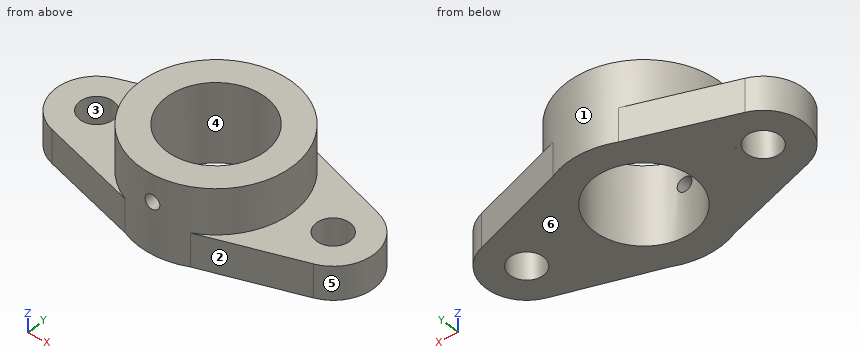
Autodesk Inventor part; units mm, degrees
ref_plane "YZ Plane" through (0, 0, 0) normal (1, 0, 0) x (0, 1, 0)
ref_plane "XZ Plane" through (0, 0, 0) normal (0, 1, 0) x (-1, 0, 0)
ref_plane "XY Plane" through (0, 0, 0) normal (0, 0, 1) x (1, 0, 0)
sketch "Boceto1" plane through (0, 0, 0) normal (0, 0, 1) x (1, 0, 0)
  circle A0 centre (-27.7266, -0.9426) radius 7
  circle A1 centre (-20, 3.239) radius 0.1677
  circle A2 centre (68.2698, -0.1077) radius 7
  arc A3 (73.4655, -16.2943) -> (73.5445, 16.0533) centre (68.2698, -0.1077) ccw
  circle A4 centre (20.2642, 0) radius 32
  line L0 (-33.3043, 15.1163) -> (6.9422, 29.0951)
  line L1 (73.5445, 16.0533) -> (33.5861, 29.0951)
  line L2 (-33.0105, -17.1059) -> (6.9422, -29.0951)
  line L3 (73.4655, -16.2943) -> (33.5861, -29.0951)
  arc A5 (-33.3043, 15.1163) -> (-32.6128, -17.2252) centre (-27.7266, -0.9426) ccw
  point P0 (0, 0)
  dimension "d0" = 14
  dimension "d2" = 14
  dimension "d3" = 96
  dimension "d5" = 34
  dimension "d6" = 64
  dimension "d7" = 48
extrude "Extrusión1" add sketch "Boceto1" along normal blind 14 contours L3 A4 L1 A3 | L2 A5 L0 A4
extrude "Extrusión3" add sketch "Boceto1" along normal blind 33 contours A4
sketch "Boceto4" plane through (20.2642, 0, 33) normal (0, 0, 1) x (1, 0, 0)
  circle A0 centre (0, 0) radius 20.64
  point P0 (-20.2642, 0)
  dimension "d21" = 41.28
extrude "Extrusión4" cut sketch "Boceto4" against normal through all
sketch "Boceto5" plane through (0, 0, 0) normal (0, 1, 0) x (-1, 0, 0)
  line L0 (-40.9042, 33) -> (0.3758, 33)
  line L1 (0.3758, 0) -> (-40.9042, 0)
  line L2 (-40.9042, 33) -> (0.3758, 33)
  line L3 (0.3758, 0) -> (-40.9042, 0)
  line L4 (-40.9042, 33) -> (0.3758, 33)
  line L5 (0.3758, 0) -> (-40.9042, 0)
  line L6 (-40.9042, 33) -> (0.3758, 33)
  line L7 (-20.3915, 34.6516) -> (-20.3915, 21.6516)
  line L8 (11.7358, 33) -> (-52.2642, 33)
  line L9 (-20.3915, 34.6516) -> (-7.3915, 34.6516) construction
  circle A0 centre (-20.3915, 21.6516) radius 3
  point P0 (0, 0)
  point P1 (-20.2642, 0)
  dimension "d24" = 13
  dimension "d25" = 90
  dimension "d26" = 6
extrude "Extrusión5" cut sketch "Boceto5" against normal blind 33
properties part number "Chumacera"
Design review of the part built by this model. Coordinates are the model's own, in mm. Face numbers are marked on the shaded views. A direction names the side the tool comes from. Coordinates: 2 decimals unless noted, no trailing zeros. Write each loop counter-clockwise with the first axis right and the second up, starting at its lowest first coordinate (ties: lowest second). Pieces come first, ordered by that corner, then holes. Notation, with made-up numbers: M 49.25,-25 L 75.25,-25 A11 ccw 75.25,-17 Z; hole C 11.25,-2 d4. An arc over 180 degrees is marked long. Answer as a JSON object with one key per item and string values.
Item 1: Add section C-C, the plane y = 11. Give the boundary of the cut face in (x, z).
Outcome:
{"outline": "M -39.83,0 L 2.8,0 L 2.8,33 L -9.79,33 L -9.79,14 L -39.83,14 Z; M 37.73,0 L 81.14,0 L 81.14,14 L 50.31,14 L 50.31,33 L 37.73,33 Z"}
Item 2: Machinability: for the marked faces 1 and 2, which of the approach directions +Z, -Z, +X, -X, +Y, -Y give a long, thin tool a straight path to every point of the face, cutting with its end or side? Answer none if there is none.
Outcome:
{"face 1": "+Z", "face 2": "+Z, -Z, +X, -Y"}
Item 3: Draft analysis for pull direction X (two halves, no side actions). For the marked faces 3, 4, 5 and 6, state which applies: pulls with the +X half, pulls with the -X half, needs draft (parallel to the pull), parting line crosses it, or undercut.
Outcome:
{"face 3": "undercut", "face 4": "undercut", "face 5": "pulls with the +X half", "face 6": "needs draft"}
Item 4: Add section D-D, the plane z = 29. Give the boundary of the cut face in (x, y).
Outcome:
{"outline": "C 20.26,0 d64; hole C 20.26,0 d41.28"}
Item 5: Insertion check: pin 1 Ø16 at (x, y) = (-27.73, -0.94) entering from -Z; pin 2 Ø3.5 at (x, z) = (20.39, 21.65) entering from -Y; pin 3 Ø18 at (x, y) = (68.27, -0.11) entering from +Z; pin 4 Ø3 at (y, z) = (-16, 28) entering from -X. Each pin has a flat end and moves straight along its axis. Give the tip position at first contact, or say it passes through.
Outcome:
{"pin 1": "z = 0", "pin 2": "y = 20.55", "pin 3": "z = 14", "pin 4": "x = -8.26"}
Item 6: Add section B-B, the plane z = 6. Give the boundary of the cut face in (x, y), and give its area (3 significant figures).
Outcome:
{"outline": "M -33.3,15.12 A17 ccw -32.61,-17.23 L 6.94,-29.1 A32 ccw 33.59,-29.1 L 73.47,-16.29 A17 ccw 73.54,16.05 L 33.59,29.1 A32 ccw 6.94,29.1 Z; hole C -27.73,-0.94 d14; hole C -20,3.24 d0.34; hole C 20.26,0 d41.28; hole C 68.27,-0.11 d14", "area": "4,180 mm²"}
Item 7: Wall thickness on probe 1 along X at (y, z) = (-4, 10); probe 2 along Z at (x, y) = (47.5, -21); probe 3 along X at (y, z) = (-4, 23.5): over which ranges is each line inside the solid? List them lowest first.
Outcome:
{"probe 1": "-44.45 to -34.02, -21.43 to 0.02, 40.51 to 62.45, 74.09 to 84.82", "probe 2": "0 to 14", "probe 3": "-11.48 to 0.02, 40.51 to 52.01"}
Item 8: Add section A-A, the plane x = 8.5. Give the boundary of the cut face in (y, z), and give its area (3 significant figures).
Outcome:
{"outline": "M -29.76,0 L -16.96,0 L -16.96,33 L -29.76,33 Z; M 16.96,0 L 29.76,0 L 29.76,33 L 16.96,33 Z", "area": "845 mm²"}
